Geometry: final body of the model. Coordinates: model frame, mm. A direction names the side the tool comes from. Round coordinates to 2 decimals unless told otherwise and drop trailing zeros. Loops run counter-clockwise (first coordinate to the right, second up) from the corner with the lowest first, then second, coordinate; pieces in that order, holes last. Notation, with made-up numbers: (88.5, 70.25) -> (106.5, 70.25) arc R30 cw to (106.5, 104.25) -> close; hole circle Ø8 at (39, 35). An arc over 180 degrees is marked (long way). Answer in a Markdown table with one row per item.
```python
from build123d import *

# Parameters (mm, degrees)
SKETCH_1_R          = 68
SKETCH_1_R_2        = 5.5
EXTRUDE_1_DEPTH     = 60
SKETCH_2_R          = 8.75
CUT_EXTRUDE_1_DEPTH = 10.8
SKETCH_4_R          = 8.75
CUT_EXTRUDE_2_DEPTH = 10.8
SKETCH_5_R          = 68
CUT_EXTRUDE_3_DEPTH = 38
SKETCH_11_R         = 1
CUT_EXTRUDE_4_DEPTH = 99.650899641


with BuildPart() as part:
    # Sketch 1 → Extrude 1 (new body)
    with BuildSketch(Plane(origin=(0, 0, 0), x_dir=(1, 0, 0), z_dir=(0, 1, 0))):
        with Locations(Location((0, 0, 0), (0, 0, 270))):
            Circle(SKETCH_1_R)
        with Locations(Location((0, 57, 0), (0, 0, 270))):
            Circle(SKETCH_1_R_2, mode=Mode.SUBTRACT)
        with Locations(Location((28.5, 49.363448016, 0), (0, 0, 270))):
            Circle(SKETCH_1_R_2, mode=Mode.SUBTRACT)
        with Locations(Location((49.363448016, 28.5, 0), (0, 0, 270))):
            Circle(SKETCH_1_R_2, mode=Mode.SUBTRACT)
        with Locations(Location((57, 0, 0), (0, 0, 270))):
            Circle(SKETCH_1_R_2, mode=Mode.SUBTRACT)
        with Locations(Location((49.363448016, -28.5, 0), (0, 0, 270))):
            Circle(SKETCH_1_R_2, mode=Mode.SUBTRACT)
        with Locations(Location((28.5, -49.363448016, 0), (0, 0, 270))):
            Circle(SKETCH_1_R_2, mode=Mode.SUBTRACT)
        with Locations(Location((0, -57, 0), (0, 0, 270))):
            Circle(SKETCH_1_R_2, mode=Mode.SUBTRACT)
        with Locations(Location((-28.5, -49.363448016, 0), (0, 0, 270))):
            Circle(SKETCH_1_R_2, mode=Mode.SUBTRACT)
        with Locations(Location((-49.363448016, -28.5, 0), (0, 0, 270))):
            Circle(SKETCH_1_R_2, mode=Mode.SUBTRACT)
        with Locations(Location((-57, 0, 0), (0, 0, 270))):
            Circle(SKETCH_1_R_2, mode=Mode.SUBTRACT)
        with Locations(Location((-49.363448016, 28.5, 0), (0, 0, 270))):
            Circle(SKETCH_1_R_2, mode=Mode.SUBTRACT)
        with Locations(Location((-28.5, 49.363448016, 0), (0, 0, 270))):
            Circle(SKETCH_1_R_2, mode=Mode.SUBTRACT)
    extrude(amount=EXTRUDE_1_DEPTH)

    # Sketch 2 → Cut-Extrude 1 (cut)
    with BuildSketch(Plane(origin=(0, 60, 0), x_dir=(1, 0, 0), z_dir=(0, 1, 0))):
        with Locations(Location((0, 57, 0), (0, 0, 270))):
            Circle(SKETCH_2_R)
        with Locations(Location((49.363448016, 28.5, 0), (0, 0, 270))):
            Circle(SKETCH_2_R)
        with Locations(Location((49.363448016, -28.5, 0), (0, 0, 270))):
            Circle(SKETCH_2_R)
        with Locations(Location((0, -57, 0), (0, 0, 270))):
            Circle(SKETCH_2_R)
        with Locations(Location((-49.363448016, -28.5, 0), (0, 0, 270))):
            Circle(SKETCH_2_R)
        with Locations(Location((-49.363448016, 28.5, 0), (0, 0, 270))):
            Circle(SKETCH_2_R)
    extrude(amount=-CUT_EXTRUDE_1_DEPTH, mode=Mode.SUBTRACT)

    # Sketch 4 → Cut-Extrude 2 (cut)
    with BuildSketch(Plane.XZ):
        with Locations(Location((28.5, 49.363448016, 0), (0, 0, 270))):
            Circle(SKETCH_4_R)
        with Locations(Location((57, 0, 0), (0, 0, 270))):
            Circle(SKETCH_4_R)
        with Locations(Location((28.5, -49.363448016, 0), (0, 0, 270))):
            Circle(SKETCH_4_R)
        with Locations(Location((-28.5, -49.363448016, 0), (0, 0, 270))):
            Circle(SKETCH_4_R)
        with Locations(Location((-57, 0, 0), (0, 0, 270))):
            Circle(SKETCH_4_R)
        with Locations(Location((-28.5, 49.363448016, 0), (0, 0, 270))):
            Circle(SKETCH_4_R)
    extrude(amount=-CUT_EXTRUDE_2_DEPTH, mode=Mode.SUBTRACT)

    # Sketch 5 → Cut-Extrude 3 (cut)
    with BuildSketch(Plane.XZ):
        with Locations(Location((0, 0, 0), (0, 0, 270))):
            Circle(SKETCH_5_R)
    extrude(amount=-CUT_EXTRUDE_3_DEPTH, mode=Mode.SUBTRACT)

    # Sketch 10 → Cut-Revolve 6 (revolve, cut)
    with BuildSketch(Plane(origin=(0, 0, 0), x_dir=(-1, 0, 0), z_dir=(0, 0, -1))):
        with BuildLine():
            Line((0, 86.414873748), (0, -10.414873748))
            ThreePointArc((0, -10.414873748), (-48.414873748, 38), (0, 86.414873748))
        make_face()
    revolve(axis=Axis((0, 86.414873748, 0), (0, -1, 0)), mode=Mode.SUBTRACT)

    # Sketch 11 → Cut-Extrude 4 (cut, through all)
    with BuildSketch(Plane(origin=(0, 60, 0), x_dir=(1, 0, 0), z_dir=(0, 1, 0))):
        with Locations(Location((15.529142706, 57.955549577, 0), (0, 0, 270))):
            Circle(SKETCH_11_R)
        with Locations(Location((42.426406871, 42.426406871, 0), (0, 0, 270))):
            Circle(SKETCH_11_R)
        with Locations(Location((57.955549577, 15.529142706, 0), (0, 0, 270))):
            Circle(SKETCH_11_R)
        with Locations(Location((57.955549577, -15.529142706, 0), (0, 0, 270))):
            Circle(SKETCH_11_R)
        with Locations(Location((42.426406871, -42.426406871, 0), (0, 0, 270))):
            Circle(SKETCH_11_R)
        with Locations(Location((15.529142706, -57.955549577, 0), (0, 0, 270))):
            Circle(SKETCH_11_R)
        with Locations(Location((-15.529142706, -57.955549577, 0), (0, 0, 270))):
            Circle(SKETCH_11_R)
        with Locations(Location((-42.426406871, -42.426406871, 0), (0, 0, 270))):
            Circle(SKETCH_11_R)
        with Locations(Location((-57.955549577, -15.529142706, 0), (0, 0, 270))):
            Circle(SKETCH_11_R)
        with Locations(Location((-57.955549577, 15.529142706, 0), (0, 0, 270))):
            Circle(SKETCH_11_R)
        with Locations(Location((-42.426406871, 42.426406871, 0), (0, 0, 270))):
            Circle(SKETCH_11_R)
        with Locations(Location((-15.529142706, 57.955549577, 0), (0, 0, 270))):
            Circle(SKETCH_11_R)
    extrude(amount=-CUT_EXTRUDE_4_DEPTH, mode=Mode.SUBTRACT)


solid = part.part
```
Item 1: First-contact query: P1, Ø12, axis at y = 46, z = -22.5, coming from the +X side; P2, Ø10, axis at y = 42, z = 1, coming from the +X side; P3, Ø6, axis at x = 27, y = 42, coming from the -Z side. Flat tips, straight axial feed; report the tip coordinate or a pass-through.
Ans:
| item | result |
|---|---|
| P1 | x = 65.97 |
| P2 | x = 68 |
| P3 | z = -63.62 |
Item 2: Set-up query: faces 4 (the cylindrical face through (-43.91, 43.52, -29.22)), 5 (the cylindrical face through (58.04, 54.68, 27.36)). Return all of +Z, -Z, +X, -X, +Y, -Y with unobstructed straight access to the full face (end or side cutting, diameter ignored); none if empty.
Ans:
| item | result |
|---|---|
| face 4 | +Y, -Y |
| face 5 | +Y |
Item 3: Section query D-D, the plane z = 12. Output: boundary loops of the cut face in (x, y), and give its area (3 significant figures).
Ans:
| item | result |
|---|---|
| outline | (-66.93, 38) -> (-46.9, 38) arc R46.9 cw to (-41.42, 60) -> (-66.93, 60) -> close; (41.42, 60) arc R46.9 cw to (46.9, 38) -> (66.93, 38) -> (66.93, 60) -> close |
| area | 960 mm2 |
Item 4: Mould query, pull axis X, two halves, no side actions, for faces 1 (the cylindrical face through (67.42, 48.85, -8.85)), 2 (the flat face through (20, 38, -45)), 3 (the flat face through (-53, 49.2, -33)). Classes: released by +X, released by -X, zero draft, split by the parting line, or undercut.
Ans:
| item | result |
|---|---|
| face 1 | split by the parting line |
| face 2 | zero draft |
| face 3 | undercut |
Item 5: Section query C-C, the plane x = 38. Output: boundary loops of the cut face in (y, z).
Ans:
| item | result |
|---|---|
| outline | (38, -56.39) -> (60, -56.39) -> (60, -20.4) arc R30 cw to (38, -30) -> close; (38, 30) arc R30 cw to (60, 20.4) -> (60, 56.39) -> (38, 56.39) -> close |
Item 6: Section query A-A, the plane z = 29. Output: boundary loops of the cut face in (x, y), and give its area (3 significant figures).
Ans:
| item | result |
|---|---|
| outline | (-61.51, 38) -> (-54.84, 38) -> (-54.84, 49.2) -> (-58.1, 49.2) -> (-58.1, 60) -> (-61.51, 60) -> close; (-43.89, 38) -> (-38.77, 38) arc R38.77 cw to (-31.92, 60) -> (-40.63, 60) -> (-40.63, 49.2) -> (-43.89, 49.2) -> close; (31.92, 60) arc R38.77 cw to (38.77, 38) -> (43.89, 38) -> (43.89, 49.2) -> (40.63, 49.2) -> (40.63, 60) -> close; (54.84, 38) -> (61.51, 38) -> (61.51, 60) -> (58.1, 60) -> (58.1, 49.2) -> (54.84, 49.2) -> close |
| area | 474 mm2 |
Item 7: Ray query, L1, parallel to X at y = 54.75, z = -28.5; L2, parallel to X at y = 43.5, z = -28.5; L3, parallel to Z at x = -24, y = 59.25. Return the intervals inside material, ascending.
Ans:
| item | result |
|---|---|
| L1 | -61.74 to -58.11, -40.61 to -35.37, 35.37 to 40.61, 58.11 to 61.74 |
| L2 | -61.74 to -54.86, -43.86 to -38.75, 38.75 to 43.86, 54.86 to 61.74 |
| L3 | -63.62 to -52.53, -46.2 to -36.28, 36.28 to 46.2, 52.53 to 63.62 |
Item 8: Section query B-B, the plane y = 57.25. State how many separate pieces and enclosed holes the cut face has, and give its area (3 significant figures).
Ans:
| item | result |
|---|---|
| separate pieces | 1 |
| enclosed holes | 25 |
| area | 6,280 mm2 |
